Work out the finished part from the listing and answer in its coordinate system (mm). Face numbers are marked on the shaded views. A direction names the side the tool comes from. Give positions to 0.01 mm unless a question says otherwise; leave off trailing zeros. Loops run counter-clockwise (first coordinate to the right, second up) from the corner with the lowest first, then second, coordinate; pieces in that order, holes last.
from build123d import *

# Parameters (mm, degrees)
PAD_DEPTH    = 100
SKETCH001_R  = 2
POCKET_DEPTH = 25.001
FILLET_R     = 3


with BuildPart() as part:
    # Sketch → Pad (new body)
    with BuildSketch(Plane.XZ):
        with BuildLine():
            Line((-6.175, 0), (-6.175, 12.225))
            ThreePointArc((6.175, 12.225), (0, 18.4), (-6.175, 12.225))
            Line((6.175, 12.225), (6.175, 0))
            Line((6.175, 0), (12.5, 0))
            Line((12.5, 0), (12.5, 12.225))
            ThreePointArc((12.5, 12.225), (0, 24.725), (-12.5, 12.225))
            Line((-12.5, 0), (-12.5, 12.225))
            Line((-12.5, 0), (-6.175, 0))
        make_face()
    extrude(amount=PAD_DEPTH)

    # Sketch001 (on Face6 of Pad) → Pocket (cut, through all)
    with BuildSketch(Plane(origin=(12.5, 0, 0), x_dir=(0, 0, 1), z_dir=(1, 0, 0))):
        with Locations((6.1125, 10)):
            Circle(SKETCH001_R)
        with Locations((6.1125, 90)):
            Circle(SKETCH001_R)
        with Locations((6.1125, 70)):
            Circle(SKETCH001_R)
        with Locations((6.1125, 30)):
            Circle(SKETCH001_R)
    extrude(amount=-POCKET_DEPTH, mode=Mode.SUBTRACT)

    # Fillet
    fillet_edges = [part.edges().sort_by_distance(p)[0] for p in [
        (12.5, -50, 0),
        (-12.5, -50, 0),
    ]]
    fillet(fillet_edges, radius=FILLET_R)


solid = part.part
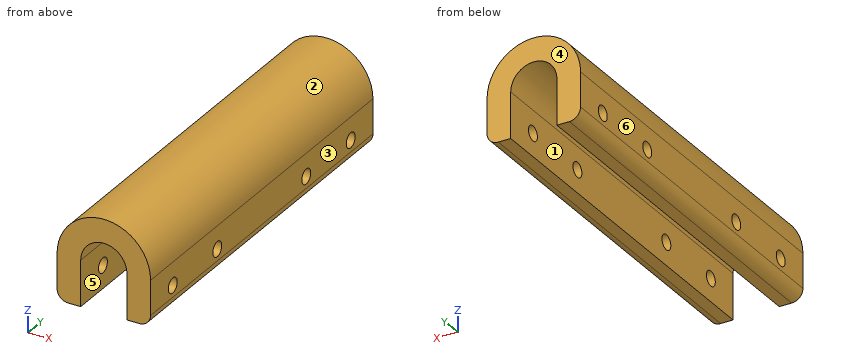
Item 1: Find section A-A, the plane y = -90. Give the number of separate pieces and of enclosed holes in the cut face, plus the area to 3 significant figures.
Item 2: Flat-ended cylindrical pins translate along their axes: pin 1 Ø3.5 at (y, z) = (-30, 6.11) entering from -X; pin 2 Ø2 at (y, z) = (-74.5, 17.5) entering from +X; pin 3 Ø3 at (y, z) = (-49.5, 16) entering from -X; pin 4 Ø5 at (y, z) = (-66, 18) entering from +X. Find the tip coordinate at first contact, or state that the pin passes through.
Item 3: Find section C-C, the plane x = 0. Write down the section's boundary in (y, z) (3 decimals), plus the area to 4 significant figures.
Item 4: Find section B-B, the plane y = -59. Write down the section's boundary in (x, z) (3 decimals), plus the area to 3 significant figures.
Item 5: For the marked faces 1 and 2, determine the directions among +Z, -Z, +X, -X, +Y, -Y from which every point of the face is accessible in a straight line to the end or side of a thin tool.
Item 6: Determine the mould class of the marked faces 3, 4, 5 and 6 for opening direction X: released by +X, released by -X, zero draft, split by the parting line, or undercut.
Item 7: Consider line 1 (X direction, y = -39.5, z = 4.75) (3 decimals); line 2 (Y direction, x = 9, z = 5.5); line 3 (Z direction, x = 10, y = -10) (1 decimal). Determine where each line is inside the solid, lowest interval first.
Ans:
1. separate pieces: 3
1. enclosed holes: 0
1. area: 286 mm2
2. pin 1: passes through
2. pin 2: stops at x = 11.75
2. pin 3: stops at x = -12.29
2. pin 4: stops at x = 12.06
3. outline: (-100, 18.4) - (0, 18.4) - (0, 24.725) - (-100, 24.725) - close
3. area: 632.5 mm2
4. outline: (-12.5, 3) arc R3 ccw to (-9.5, 0) - (-6.175, 0) - (-6.175, 12.225) arc R6.175 cw to (6.175, 12.225) - (6.175, 0) - (9.5, 0) arc R3 ccw to (12.5, 3) - (12.5, 12.225) arc R12.5 ccw to (-12.5, 12.225) - close
4. area: 336 mm2
5. face 1: -Z, +Y, -Y
5. face 2: +Z, +Y, -Y
6. face 3: released by +X
6. face 4: zero draft
6. face 5: undercut
6. face 6: released by -X
7. line 1: x = -12.5 to -6.175, 6.175 to 12.5
7. line 2: y = -100 to -91.9, -88.1 to -71.9, -68.1 to -31.9, -28.1 to -11.9, -8.1 to 0
7. line 3: z = 0 to 4.1, 8.1 to 19.7
